Here's how the part is built. I have some questions about the finished solid (model axes, mm). Coordinates: 2 decimals unless noted, no trailing zeros. Write each loop counter-clockwise with the first axis right and the second up, starting at its lowest first coordinate (ties: lowest second). Pieces come first, ordered by that corner, then holes.
Item 1: If we section it at B-B (y = 16.25): Please give me the cut outline in (x, z) (3 decimals), then the cut area to 3 significant figures.
Item 2: If we section it at A-A (z = 94.5): Please give me the cut outline in (x, y) (3 decimals), then the cut area to 3 significant figures.
Item 3: If I drill on line 1 (X direction, y = 1.25, z = 368.3) (3 decimals); line 2 (X direction, y = 1.75, z = 457.2) (3 decimals); line 3 (Y direction, x = 25.5, z = 108) (3 decimals), over which ranges is the centre line in solid material (lowest first)?
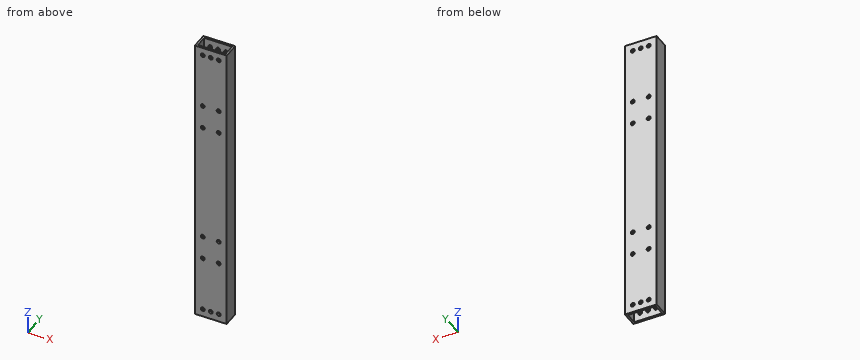
from build123d import *

# Parameters (mm, degrees)
SKETCH1_W               = 50.8
SKETCH1_H               = 25.4
SKETCH1_W_2             = 44.45
SKETCH1_H_2             = 19.05
BOSS_EXTRUDE1_DEPTH     = 469.9
CUT_EXTRUDE1_DEPTH      = 474.319986901
CUT_EXTRUDE1_DEPTH_BACK = 474.319986901
SKETCH3_R               = 3.175
CUT_EXTRUDE2_DEPTH      = 474.319986901
CUT_EXTRUDE2_DEPTH_BACK = 474.319986901
SKETCH4_R               = 3.175


with BuildPart() as part:
    # Sketch1 → Boss-Extrude1 (new body)
    with BuildSketch(Plane.XY):
        with Locations((25.4, 12.7)):
            Rectangle(SKETCH1_W, SKETCH1_H)
        with Locations((25.4, 12.7)):
            Rectangle(SKETCH1_W_2, SKETCH1_H_2, mode=Mode.SUBTRACT)
    extrude(amount=BOSS_EXTRUDE1_DEPTH)

    # Sketch3 → Cut-Extrude1 (cut, two sides: drawn at the far end of the back side and taken through both)
    with BuildSketch(Plane(origin=(0, 25.4, 0), x_dir=(1, 0, 0), z_dir=(0, 1, 0)).offset(-CUT_EXTRUDE1_DEPTH_BACK)):
        with Locations(Location((12.7, -12.7, 0), (0, 0, 270))):
            Circle(SKETCH3_R)
        with Locations(Location((12.7, -457.2, 0), (0, 0, 270))):
            Circle(SKETCH3_R)
        with Locations(Location((25.4, -457.2, 0), (0, 0, 270))):
            Circle(SKETCH3_R)
        with Locations(Location((25.4, -12.7, 0), (0, 0, 270))):
            Circle(SKETCH3_R)
        with Locations(Location((38.1, -457.2, 0), (0, 0, 270))):
            Circle(SKETCH3_R)
        with Locations(Location((38.1, -12.7, 0), (0, 0, 270))):
            Circle(SKETCH3_R)
    extrude(amount=CUT_EXTRUDE1_DEPTH + CUT_EXTRUDE1_DEPTH_BACK, mode=Mode.SUBTRACT)

    # Sketch4 → Cut-Extrude2 (cut, two sides: drawn at the far end of the back side and taken through both)
    with BuildSketch(Plane(origin=(0, 25.4, 0), x_dir=(1, 0, 0), z_dir=(0, 1, 0)).offset(-CUT_EXTRUDE2_DEPTH_BACK)):
        with Locations(Location((12.7, -139.7, 0), (0, 0, 90))):
            Circle(SKETCH4_R)
        with Locations(Location((12.7, -330.2, 0), (0, 0, 90))):
            Circle(SKETCH4_R)
        with Locations(Location((12.7, -101.6, 0), (0, 0, 90))):
            Circle(SKETCH4_R)
        with Locations(Location((12.7, -368.3, 0), (0, 0, 90))):
            Circle(SKETCH4_R)
        with Locations(Location((38.1, -101.6, 0), (0, 0, 90))):
            Circle(SKETCH4_R)
        with Locations(Location((38.1, -139.7, 0), (0, 0, 90))):
            Circle(SKETCH4_R)
        with Locations(Location((38.1, -330.2, 0), (0, 0, 90))):
            Circle(SKETCH4_R)
        with Locations(Location((38.1, -368.3, 0), (0, 0, 90))):
            Circle(SKETCH4_R)
    extrude(amount=CUT_EXTRUDE2_DEPTH + CUT_EXTRUDE2_DEPTH_BACK, mode=Mode.SUBTRACT)


solid = part.part
Answer list:
1. outline: (0, 0) - (3.175, 0) - (3.175, 469.9) - (0, 469.9) - close; (47.625, 0) - (50.8, 0) - (50.8, 469.9) - (47.625, 469.9) - close
1. area: 2,980 mm2
2. outline: (0, 0) - (50.8, 0) - (50.8, 25.4) - (0, 25.4) - close; hole (3.175, 3.175) - (47.625, 3.175) - (47.625, 22.225) - (3.175, 22.225) - close
2. area: 444 mm2
3. line 1: x = 0 to 9.525, 15.875 to 34.925, 41.275 to 50.8
3. line 2: x = 0 to 9.525, 15.875 to 22.225, 28.575 to 34.925, 41.275 to 50.8
3. line 3: y = 0 to 3.175, 22.225 to 25.4
